```python
from build123d import *

# Parameters (mm, degrees)
BOSS_EXTRUDE1_DEPTH     = 15
BOSS_EXTRUDE2_DEPTH     = 2
CUT_EXTRUDE1_DEPTH      = 10.15
CUT_EXTRUDE2_DEPTH      = 4.85
CUT_EXTRUDE5_DEPTH      = 37.462309307
CUT_EXTRUDE5_DEPTH_BACK = 37.462309307
CHAMFER3_SIZE           = 2
CUT_EXTRUDE6_DEPTH      = 60.299036748
CUT_EXTRUDE6_DEPTH_BACK = 60.299036748
SKETCH6_W               = 39.703071578
SKETCH6_H               = 42.363425718


with BuildPart() as part:
    # Sketch1 → Boss-Extrude1 (new body)
    with BuildSketch(Plane(origin=(0, 0, 0), x_dir=(1, 0, 0), z_dir=(0, 1, 0))):
        Polygon((23.5, 9.391735838), (-5, 9.391735838), (-5, -4.108264162), (10, -4.108264162), (10, -19.108264162), (23.5, -19.108264162), align=None)
        Polygon((0, 4.391735838), (0, 0.891735838), (15, 0.891735838), (15, -14.108264162), (18.5, -14.108264162), (18.5, 4.391735838), align=None, mode=Mode.SUBTRACT)
    extrude(amount=BOSS_EXTRUDE1_DEPTH)

    # Sketch2 → Boss-Extrude2 (add)
    with BuildSketch(Plane.XZ):
        Polygon((-5, 4.108264162), (10, 4.108264162), (10, 19.108264162), (23.5, 19.108264162), (23.5, -9.391735838), (-5, -9.391735838), align=None)
    extrude(amount=BOSS_EXTRUDE2_DEPTH)

    # Sketch3 → Cut-Extrude1 (cut)
    with BuildSketch(Plane(origin=(0, 15, 0), x_dir=(1, 0, 0), z_dir=(0, 1, 0))):
        Polygon((18.5, 4.391735838), (-5, 4.391735838), (-5, 0.891735838), (-5, -4.108264162), (10, -4.108264162), (10, -19.108264162), (15, -19.108264162), (18.5, -19.108264162), align=None)
    extrude(amount=-CUT_EXTRUDE1_DEPTH, mode=Mode.SUBTRACT)

    # Sketch4 → Cut-Extrude2 (cut)
    with BuildSketch(Plane(origin=(0, 4.85, 0), x_dir=(1, 0, 0), z_dir=(0, 1, 0))):
        Polygon((-5, 4.391735838), (18.5, 4.391735838), (18.5, -19.108264162), (15, -19.108264162), (15, 0.891735838), (-5, 0.891735838), align=None)
    extrude(amount=-CUT_EXTRUDE2_DEPTH, mode=Mode.SUBTRACT)

    # Sketch5 → Cut-Extrude5 (cut, two sides: drawn at the far end of the back side and taken through both)
    with BuildSketch(Plane.XY.offset(-4.391735838).offset(-CUT_EXTRUDE5_DEPTH_BACK)):
        Polygon((-5, 4.85), (18.5, 4.85), (18.5, 8.35), (-10.741212184, 8.35), (-10.741212184, 4.85), align=None)
    extrude(amount=CUT_EXTRUDE5_DEPTH + CUT_EXTRUDE5_DEPTH_BACK, mode=Mode.SUBTRACT)

    # Chamfer3
    chamfer3_edges = [part.edges().sort_by_distance(p)[0] for p in [
        (6.75, 8.35, -9.391735838),
        (6.75, 4.85, -9.391735838),
    ]]
    chamfer(chamfer3_edges, length=CHAMFER3_SIZE)


with BuildPart() as body_2:
    # Mirror1: mirrored copy
    add(part.part.mirror(Plane.ZY.offset(15)))


with BuildPart() as part_1:
    add(part.part)

    # Sketch6 → Cut-Extrude6 (cut, two sides: drawn at the far end of the back side and taken through both)
    with BuildSketch(Plane(origin=(0, 15, 0), x_dir=(1, 0, 0), z_dir=(0, 1, 0)).offset(-CUT_EXTRUDE6_DEPTH_BACK)):
        with Locations((10, -4.108264162)):
            Rectangle(SKETCH6_W, SKETCH6_H)
    extrude(amount=CUT_EXTRUDE6_DEPTH + CUT_EXTRUDE6_DEPTH_BACK, mode=Mode.SUBTRACT)


solid = body_2.part
```
The listing builds one solid part. Answer for the finished solid, in the listing's coordinates (mm). A direction names the side the tool comes from. Give positions to 0.01 mm unless a question says otherwise; leave off trailing zeros. Order: outer loops, then holes, each group sorted by start corner. A loop starts at its lowest first (then second) coordinate and runs counter-clockwise, first axis right, second up.
1) Find section C-C on z = -5. Write down the section's boundary in (x, y).
Reported:
outline: (-53.5, -2) - (-25, -2) - (-25, 4.85) - (-48.5, 4.85) - (-48.5, 8.35) - (-25, 8.35) - (-25, 15) - (-53.5, 15) - close
2) Determine the mould class of faces 4 (the face through (-36.59, 3.86, -8.38)), 5 (the face through (-37, 2, -4.392)), 6 (the face through (-43, -2, 2)), 7 (the face through (-37, 4.85, -6)) for opening direction Y: pulls with the +Y half, pulls with the -Y half, needs draft (parallel to the pull), parting line crosses it, or undercut.
Reported:
face 4: undercut
face 5: needs draft
face 6: pulls with the -Y half
face 7: undercut
3) Find section D-D on y = 11.25. Write down the section's boundary in (x, z), then the cut area to 3 significant figures.
Reported:
outline: (-53.5, -9.39) - (-25, -9.39) - (-25, -4.39) - (-48.5, -4.39) - (-48.5, 19.11) - (-53.5, 19.11) - close
area: 260 mm2
4) Find section A-A on x = -43.5. Write down the section's boundary in (y, z).
Reported:
outline: (-2, -9.39) - (2.85, -9.39) - (4.85, -7.39) - (4.85, -4.39) - (0, -4.39) - (0, -0.89) - (4.85, -0.89) - (4.85, 19.11) - (-2, 19.11) - close; (8.35, -7.39) - (10.35, -9.39) - (15, -9.39) - (15, -4.39) - (8.35, -4.39) - close
5) Consider line 1 along Z through (x, y) = (-26.5, 2); line 2 along Y through (x, z) = (-28.75, -4.75); line 3 along X through (y, z) = (1.25, 11.5). Determine where each line is inside the solid, lowest interval first.
Reported:
line 1: z = -9.39 to -4.39, -0.89 to 4.11
line 2: y = -2 to 4.85, 8.35 to 15
line 3: x = -53.5 to -48.5, -45 to -40
6) For faces 1 (the face through (-37, 12, -4.392)), 2 (the face through (-36.91, 9.34, -8.38)), 3 (the face through (-35, 2, -0.892)), determine the directions among +Z, -Z, +X, -X, +Y, -Y from which every point of the face is accessible in a straight line to the end or side of a thin tool.
Reported:
face 1: +Z, +X, +Y
face 2: -Z, +X
face 3: +X, +Y
7) Given P1, Ø7.5, axis at x = -39, y = 11, coming from the +Z side; P2, Ø1.5, axis at x = -38, y = 1, coming from the +Z side; P3, Ø10, axis at x = -33, z = 7, coming from the +Y side, each flat-ended and moving along its own axis, determine where each tip first touches the part or whether it passes through.
Reported:
P1: stops at z = -4.39
P2: stops at z = 4.11
P3: stops at y = 4.85
8) Find section B-B on y = 1.25. Write down the section's boundary in (x, z).
Reported:
outline: (-53.5, -9.39) - (-25, -9.39) - (-25, -4.39) - (-48.5, -4.39) - (-48.5, 19.11) - (-53.5, 19.11) - close; (-45, -0.89) - (-25, -0.89) - (-25, 4.11) - (-40, 4.11) - (-40, 19.11) - (-45, 19.11) - close
